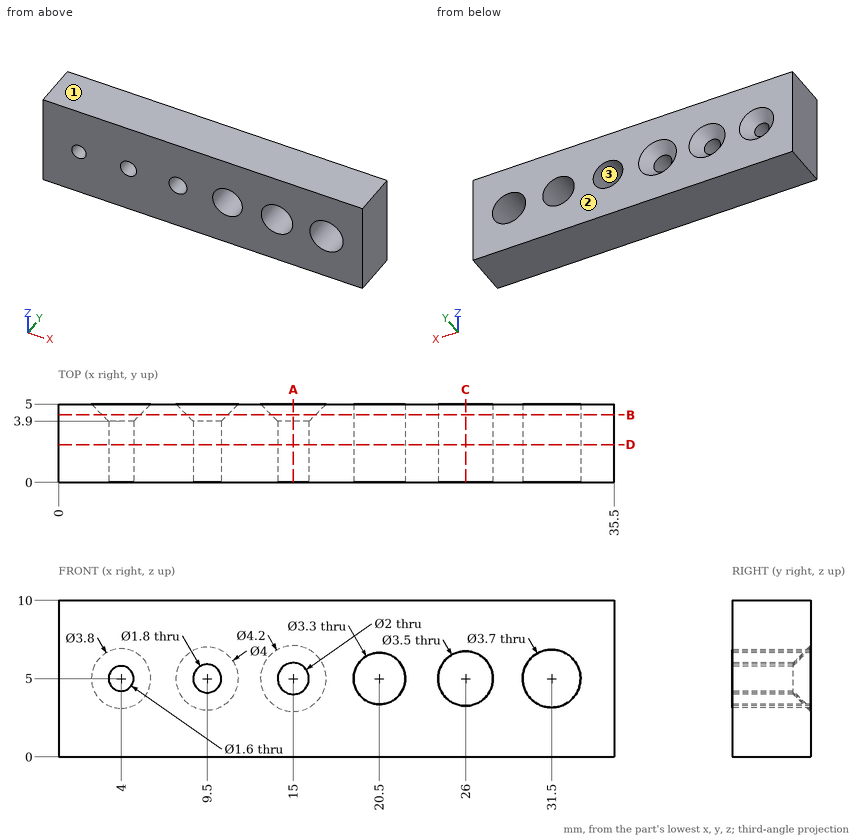
Geometry check sheet. Reference: drawing and pictorial views, mm from the part's lowest x, y, z. Coordinates: 2 decimals unless noted, no trailing zeros. Loops run counter-clockwise (first coordinate to the right, second up) from the corner with the lowest first, then second, coordinate; pieces in that order, holes last.
1) Material ranges on probe 1 along Z at (x, y) = (26, 3.1); probe 2 along Z at (x, y) = (20.5, 3.75); probe 3 along Y at (x, z) = (4, 4), recorded low to high.
2) Gauge pin test, flat end, axial feed: pin 1 (1.8 mm diameter, centred on x = 4, z = 5, fed in from +Y). Record the tip position at first contact, or that the pin passes through.
3) Sectioned sample at D-D (y = 2.4). Record the boundary of the cut face in (x, z), and give its area (3 significant figures).
4) Sectioned sample at A-A (x = 15). Record the boundary of the cut face in (y, z).
5) Sectioned sample at B-B (y = 4.3). Record the boundary of the cut face in (x, z), and give its area (3 significant figures).
6) Sectioned sample at C-C (x = 26). Record the boundary of the cut face in (y, z).
7) Release check for a two-part mould opening along Z. For the marked faces 1, 2 and 3 record: released by +Z, released by -Z, zero draft, split by the parting line, or undercut.
Check sheet entries:
1. probe 1: z = 0 to 3.25, 6.75 to 10
1. probe 2: z = 0 to 3.35, 6.65 to 10
1. probe 3: y = 0 to 4.1
2. pin 1: stops at y = 4
3. outline: (0, 0) - (35.5, 0) - (35.5, 10) - (0, 10) - close; hole circle Ø1.6 at (4, 5); hole circle Ø1.8 at (9.5, 5); hole circle Ø2 at (15, 5); hole circle Ø3.3 at (20.5, 5); hole circle Ø3.5 at (26, 5); hole circle Ø3.7 at (31.5, 5)
3. area: 318 mm2
4. outline: (0, 0) - (5, 0) - (5, 2.9) - (3.9, 4) - (0, 4) - close; (0, 6) - (3.9, 6) - (5, 7.1) - (5, 10) - (0, 10) - close
5. outline: (0, 0) - (35.5, 0) - (35.5, 10) - (0, 10) - close; hole circle Ø2.4 at (4, 5); hole circle Ø2.6 at (9.5, 5); hole circle Ø2.8 at (15, 5); hole circle Ø3.3 at (20.5, 5); hole circle Ø3.5 at (26, 5); hole circle Ø3.7 at (31.5, 5)
5. area: 310 mm2
6. outline: (0, 0) - (5, 0) - (5, 3.25) - (0, 3.25) - close; (0, 6.75) - (5, 6.75) - (5, 10) - (0, 10) - close
7. face 1: released by +Z
7. face 2: zero draft
7. face 3: undercut
